Geometry check sheet. Reference: the model listing, model coordinates, mm. A direction names the side the tool comes from. Round coordinates to 2 decimals unless told otherwise and drop trailing zeros. Order: outer loops, then holes, each group sorted by start corner. A loop starts at its lowest first (then second) coordinate and runs counter-clockwise, first axis right, second up. Notation, with made-up numbers: (26, 7.5) - (75, 7.5) arc R4 ccw to (75, 13.5) - close; hole circle Ø7 at (59, -28.5). An arc over 180 degrees is marked (long way). Write each question's results on one line, items separated by ' | '.
```python
from build123d import *

# Parameters (mm, degrees)
SKETCH1_W           = 21.59
SKETCH1_H           = 157.1752
BOSS_EXTRUDE1_DEPTH = 3.175
SKETCH2_W           = 21.59
SKETCH2_H           = 131.7752
BOSS_EXTRUDE2_DEPTH = 7.9248
SKETCH3_R           = 1.5875
CUT_EXTRUDE1_DEPTH  = 4.7752


with BuildPart() as part:
    # Sketch1 → Boss-Extrude1 (new body)
    with BuildSketch(Plane.XY):
        Rectangle(SKETCH1_W, SKETCH1_H)
    extrude(amount=BOSS_EXTRUDE1_DEPTH)

    # Sketch2 → Boss-Extrude2 (add)
    with BuildSketch(Plane(origin=(0, 0, 0), x_dir=(-1, 0, 0), z_dir=(0, 0, -1))):
        Rectangle(SKETCH2_W, SKETCH2_H)
    extrude(amount=BOSS_EXTRUDE2_DEPTH)

    # Sketch3 → Cut-Extrude1 (cut)
    with BuildSketch(Plane.XY.offset(3.175)):
        with Locations((-7.62, 75.4126)):
            Circle(SKETCH3_R)
        with Locations((7.62, 75.4126)):
            Circle(SKETCH3_R)
        with Locations((7.62, -75.4126)):
            Circle(SKETCH3_R)
        with Locations((-7.62, -75.4126)):
            Circle(SKETCH3_R)
    extrude(amount=-CUT_EXTRUDE1_DEPTH, mode=Mode.SUBTRACT)


solid = part.part
```
(1) Access from +Z, -Z, +X, -X, +Y, -Y to the whole of each face (thin tool, end or side, straight path). Record for faces 1 (the face through (0, 1, -7.925)), 2 (the face through (0, -72, 0)).
Answers follow:
face 1: -Z, +X, -X, +Y, -Y | face 2: -Z, +X, -X, -Y
(2) Draft check along Y on faces 3 (the face through (7.413, 76.987, 1.61)), 4 (the face through (0, 65.888, -4)), 5 (the face through (0, 72, 0)). Enter one of: released by +Y, released by -Y, zero draft, split by the parting line, or undercut.
Answers follow:
face 3: undercut | face 4: released by +Y | face 5: zero draft
(3) Depth check by flat-ended pin: pin 1 Ø6.5 at (x, z) = (-5.5, -6) entering from +Y; pin 2 Ø2 at (x, z) = (5.5, -3.5) entering from -Y; pin 3 Ø4 at (x, y) = (-4.5, -69.5) entering from -Z. Enter the tip coordinate at first touch or a pass-through.
Answers follow:
pin 1: y = 65.89 | pin 2: y = -65.89 | pin 3: z = 0
(4) Section check C-C (z = -4). Record the cut outline in (x, y) (3 decimals), then the cut area to 3 significant figures.
Answers follow:
outline: (-10.795, -65.888) - (10.795, -65.888) - (10.795, 65.888) - (-10.795, 65.888) - close | area: 2,850 mm²
(5) Section check A-A (x = -7.62). Record the cut outline in (y, z) (3 decimals), then the cut area to 3 significant figures.
Answers follow:
outline: (-78.588, 0) - (-77, 0) - (-77, 3.175) - (-78.588, 3.175) - close; (-73.825, 0) - (-65.888, 0) - (-65.888, -7.925) - (65.888, -7.925) - (65.888, 0) - (73.825, 0) - (73.825, 3.175) - (-73.825, 3.175) - close; (77, 0) - (78.588, 0) - (78.588, 3.175) - (77, 3.175) - close | area: 1,520 mm²
(6) Section check B-B (x = 2.5). Record the cut outline in (y, z) (3 decimals).
Answers follow:
outline: (-78.588, 0) - (-65.888, 0) - (-65.888, -7.925) - (65.888, -7.925) - (65.888, 0) - (78.588, 0) - (78.588, 3.175) - (-78.588, 3.175) - close
(7) Material ranges on line 1 (Y direction, x = -7.62, z = 0.85); line 2 (Y direction, x = -5.5, z = -6.25); line 3 (Z direction, x = -3.25, y = -68) (3 decimals), recorded low to high.
Answers follow:
line 1: -78.59 to -77, -73.83 to 73.83, 77 to 78.59 | line 2: -65.89 to 65.89 | line 3: 0 to 3.175
